Verification items for the finished model (mm, model axes). A direction names the side the tool comes from. Round coordinates to 2 decimals unless told otherwise and drop trailing zeros. Order: outer loops, then holes, each group sorted by start corner. A loop starts at its lowest first (then second) coordinate and runs counter-clockwise, first axis right, second up. Notation, with made-up numbers: (-20.5, 56) -> (-9.5, 56) arc R22 cw to (-9.5, 92) -> close; hole circle Ø1 at (-24, 36). An arc over 180 degrees is marked (long way). Write item = value, one per line. Start each with the question number.
from build123d import *

# Parameters (mm, degrees)
SKETCH1_W                        = 609.6
SKETCH1_H                        = 609.6
BOSS_EXTRUDE1_DEPTH              = 6.35
F_3_8_0_375_DIAMETER_HOLE1_D     = 9.525
F_3_8_0_375_DIAMETER_HOLE1_DEPTH = 11.684
F_3_8_0_375_DIAMETER_HOLE1_TIP   = 2.861598698
SKETCH4_R                        = 9.525
BOSS_EXTRUDE2_DEPTH              = 165.1


with BuildPart() as part:
    # Sketch1 → Boss-Extrude1 (new body)
    with BuildSketch(Plane(origin=(0, 0, 0), x_dir=(1, 0, 0), z_dir=(0, 1, 0))):
        Rectangle(SKETCH1_W, SKETCH1_H)
    extrude(amount=BOSS_EXTRUDE1_DEPTH)

    # 3/8 (0.375) Diameter Hole1
    with Locations(Plane(origin=(0, 6.35, 0), x_dir=(1, 0, 0), z_dir=(0, 1, 0))):
        with Locations((-63.5, -285.75), (63.5, -285.75), (-285.75, 63.5), (-285.75, -63.5), (-63.5, -180.975), (63.5, -180.975), (-180.975, -63.5), (-180.975, 63.5)):
            Hole(F_3_8_0_375_DIAMETER_HOLE1_D / 2, depth=F_3_8_0_375_DIAMETER_HOLE1_DEPTH)
            with Locations((0, 0, -(F_3_8_0_375_DIAMETER_HOLE1_DEPTH + F_3_8_0_375_DIAMETER_HOLE1_TIP / 2))):  # 118° drill point
                Cone(0, F_3_8_0_375_DIAMETER_HOLE1_D / 2, F_3_8_0_375_DIAMETER_HOLE1_TIP, mode=Mode.SUBTRACT)

    # Sketch4 → Boss-Extrude2 (add)
    with BuildSketch(Plane(origin=(0, 6.35, 0), x_dir=(1, 0, 0), z_dir=(0, 1, 0))):
        Circle(SKETCH4_R)
    extrude(amount=BOSS_EXTRUDE2_DEPTH)

    # Sketch5 → Revolve3 (revolve)
    with BuildSketch(Plane.XY):
        with BuildLine():
            Line((0, 200.025), (0, 168.275))
            ThreePointArc((0, 168.275), (-15.875, 184.15), (0, 200.025))
        make_face()
    revolve(axis=Axis((0, 599.823656089, 0), (0, -1, 0)))


solid = part.part
(1) Cross-section at A-A (x = 0). Enter the section's corners in (y, z) (3 decimals).
(2) Depth check by flat-ended pin: pin 1 (5.5 mm diameter, centred on x = -285.75, z = -63.5, fed in from +Y); pin 2 (15 mm diameter, centred on x = 63.5, z = 285.75, fed in from +Y). Enter the tip coordinate at first touch or a pass-through.
(3) Scan lines: line 1 along X through (y, z) = (1.75, 285.75); line 2 along X through (y, z) = (5.25, 63.5); line 3 along Z through (x, y) = (63.5, 3.5). Record each from-to range of solid material in increasing order. Write a range as from..to.
(4) Cross-section at C-C (z = 254). Enter the section's corners in (x, y), and give its area (3 significant figures).
(5) Cross-section at B-B (y = 112.5). Enter the section's corners in (x, z) (3 decimals), and give its area (3 significant figures).
(6) Set-up check for faces 1 (the cylindrical face through (-7.559, 87.744, 5.796)), 2 (the flat face through (-4, 0, -4)): record each of +Z, -Z, +X, -X, +Y, -Y from which the full face is reachable in a straight line by a thin tool's end or side.
(7) Cross-section at D-D (x = 239). Enter the section's corners in (y, z), and give its area (3 significant figures).
Outcome:
q1.outline = (0, -304.8) -> (6.35, -304.8) -> (6.35, -9.525) -> (171.45, -9.525) arc R15.875 ccw (long way) to (171.45, 9.525) -> (6.35, 9.525) -> (6.35, 304.8) -> (0, 304.8) -> close
q2.pin_1 = through
q2.pin_2 = 6.35
q3.line_1 = -304.8..-68.26, -58.74..58.74, 68.26..304.8
q3.line_2 = -304.8..-290.51, -280.99..-185.74, -176.21..304.8
q3.line_3 = -304.8..176.21, 185.74..280.99, 290.51..304.8
q4.outline = (-304.8, 0) -> (304.8, 0) -> (304.8, 6.35) -> (-304.8, 6.35) -> close
q4.area = 3,870 mm^2
q5.outline = circle Ø19.05 at (0, 0)
q5.area = 285 mm^2
q6.face_1 = none
q6.face_2 = +Z, -Z, +X, -X, -Y
q7.outline = (0, -304.8) -> (6.35, -304.8) -> (6.35, 304.8) -> (0, 304.8) -> close
q7.area = 3,870 mm^2
